The figure shows three views and two pictorial views of one solid part (mm, origin at its lowest corner). Answer the questions. Give positions to 0.01 mm unless a question says otherwise; leave off trailing zeros. Write each loop counter-clockwise with the first axis right and the second up, starting at its lowest first coordinate (ties: lowest second). Pieces come first, ordered by that corner, then holes. Notation, with made-up numbers: (76.25, -29) - (105.25, -29) arc R22 ccw to (105.25, 1) - close; hole circle Ø11 at (22.5, 27.25). An arc over 180 degrees is marked (long way). One line per question, with ' | ' between items. Start each with the question number.
1. A cutting plane is placed at D-D (y = 2.75). Determine the outline of the cut face in (x, z), then the cut area to 3 significant figures.
2. Find the intervals of material crossed by L1, parallel to X at y = 7.75, z = 19 (1 decimal); L2, parallel to Z at x = 20.5, y = 2.25; L3, parallel to Z at x = 28.5, y = 4 (1 decimal), in increasing order. Write a range as from..to.
3. The mould has two halves that part along Z. Classify the marked faces 1, 2 and 3: +Z half, -Z half, draft (parallel to the pull), parting line (faces both ways), or undercut.
4. A cutting plane is placed at C-C (x = 27.5). Determine the outline of the cut face in (y, z).
5. Given P1, Ø3, axis at x = 28.5, z = 5.28, coming from the -Y side; P2, Ø3, axis at y = 5, z = 25, coming from the -X side; P3, Ø2, axis at x = 29.5, y = 5, coming from the +Z side; P4, Ø1.5, axis at y = 6, z = 6.5, coming from the +X side, each flat-ended and moving along its own axis, determine where each tip first touches the part or whether it passes through.
6. A cutting plane is placed at B-B (z = 35.5). Determine the outline of the cut face in (x, y).
7. A cutting plane is placed at A-A (x = 6.5). Determine the outline of the cut face in (y, z), then the cut area to 3 significant figures.
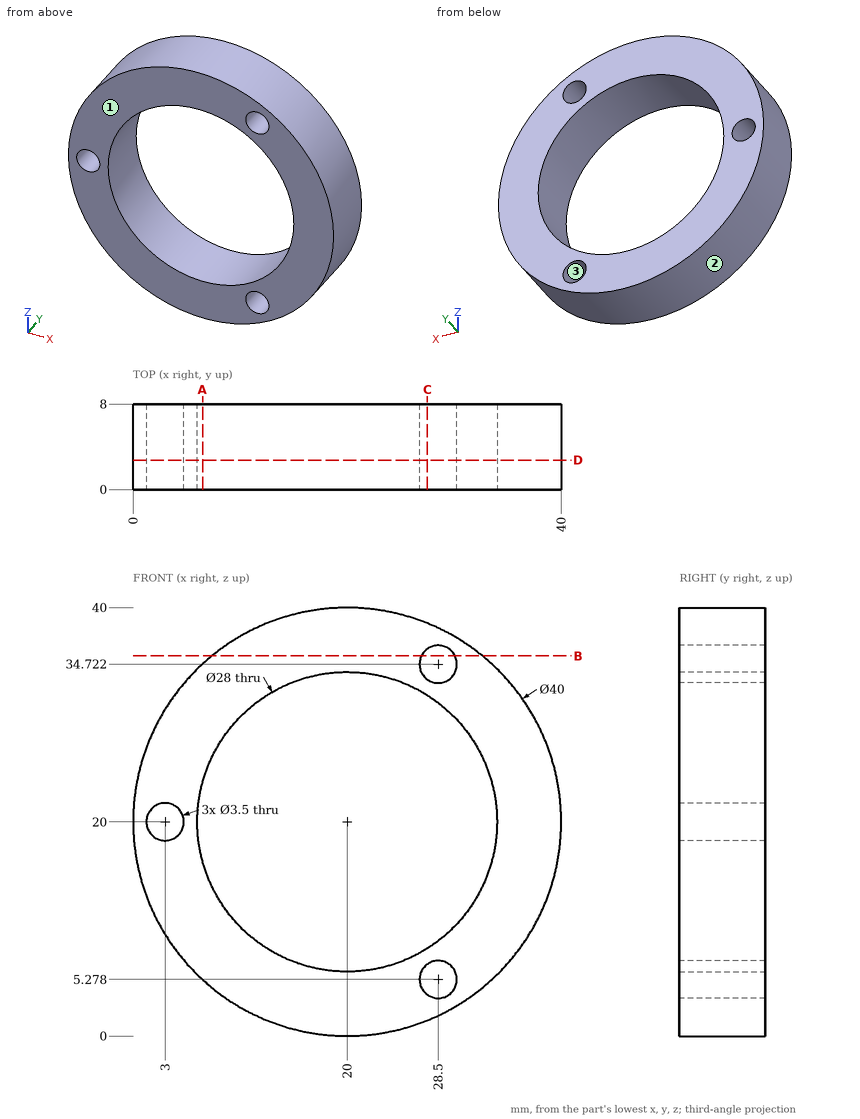
Determined:
1) outline: circle Ø40 at (20, 20); hole circle Ø3.5 at (3, 20); hole circle Ø28 at (20, 20); hole circle Ø3.5 at (28.5, 5.28); hole circle Ø3.5 at (28.5, 34.72) | area: 612 mm2
2) L1: 0..1.6, 4.4..6, 34..40 | L2: 0.01..6.01, 33.99..39.99 | L3: 1.9..3.5, 7..8.9, 31.1..33, 36.5..38.1
3) face 1: draft | face 2: parting line | face 3: undercut
4) outline: (0, 1.46) - (8, 1.46) - (8, 3.84) - (0, 3.84) - close; (0, 6.71) - (8, 6.71) - (8, 8.18) - (0, 8.18) - close; (0, 31.82) - (8, 31.82) - (8, 33.29) - (0, 33.29) - close; (0, 36.16) - (8, 36.16) - (8, 38.54) - (0, 38.54) - close
5) P1: through | P2: x = 0.31 | P3: z = 38.1 | P4: x = 35.41
6) outline: (7.36, 0) - (26.93, 0) - (26.93, 8) - (7.36, 8) - close; (30.07, 0) - (32.64, 0) - (32.64, 8) - (30.07, 8) - close
7) outline: (0, 5.24) - (8, 5.24) - (8, 16.29) - (0, 16.29) - close; (0, 23.71) - (8, 23.71) - (8, 34.76) - (0, 34.76) - close | area: 177 mm2
